Autodesk Inventor part; units mm, degrees
ref_plane "Work Plane1" through (29, 0, 0) normal (0, -1, 0) x (1, 0, 0)
ref_plane "YZ Plane" through (0, 0, 0) normal (1, 0, 0) x (0, 1, 0)
ref_plane "XZ Plane" through (0, 0, 0) normal (0, 1, 0) x (-1, 0, 0)
sketch "Sketch1" plane through (0, 0, 0) normal (0, 0, 1) x (1, 0, 0)
  line L0 (-0.5, 0) -> (6, 0)
  line L1 (6, 0) -> (6, 1)
  line L2 (6, 1) -> (1, 1)
  line L3 (1, 1) -> (0.7545, 1)
  line L4 (0.7545, 1) -> (0, 1)
  line L5 (0, 1) -> (0, 1.9)
  line L6 (0, 1.9) -> (-2, 1.9)
  line L7 (-2, 1.9) -> (-2, 0.866)
  line L8 (-2, 0.866) -> (-1, 0.866)
  line L9 (-1, 0.866) -> (-0.5, 0)
  line L10 (-3.6, 0) -> (7.6, 0)
  line L11 (0, -0.38) -> (0, 2.28)
  line L12 (1, 1) -> (0, 1) construction
  dimension "d1" = 5
  dimension "d2" = 0.2455
  dimension "d3" = 2
  dimension "d4" = 1
  dimension "d5" = 60
  dimension "d6" = 2
  dimension "d7" = 2
  dimension "d8" = 1.7321
  dimension "d9" = 3.8
  dimension "d26" = 6
revolve "Body" add sketch "Sketch1" angle 360 about axis through (-0.5, 0, 0) along (1, 0, 0)
sketch "Sketch2" plane through (-2, 0, 0) normal (-1, 0, 0) x (0, 0, 1)
  circle A0 centre (0, 0) radius 0.866
  line L0 (0, -2.66) -> (0, 2.66)
  line L1 (-2.66, 0) -> (2.66, 0)
  line L2 (0.866, 0) -> (0.433, -0.75)
  line L3 (0.433, -0.75) -> (-0.433, -0.75)
  line L4 (-0.433, -0.75) -> (-0.866, 0)
  line L5 (-0.866, 0) -> (-0.433, 0.75)
  line L6 (-0.433, 0.75) -> (0.433, 0.75)
  line L7 (0.433, 0.75) -> (0.866, 0)
  point P0 (0, 0)
extrude "Slot" add sketch "Sketch2" against normal up to next contours L7 A0 | A0 L2 | L6 L0 A0 | A0 L0 L3 | L0 L6 A0 | A0 L3 L0 | L4 A0 | A0 L5
fillet "Fillet1" radius 0.2 1 edges at (-2, -1.9, 0)
thread "Thread"
chamfer "Chamfer1" distance 0.2454 distance2 0.2454 1 edges at (6, -1, 0) measured on face at (6, -0.4588, -0.3309)
ref_plane "Work Plane1" through (29, 0, 0) normal (0, -1, 0) x (1, 0, 0)
fillet "Fillet2" radius 0.1 1 edges at (0, -1, 0)
equation "\"d1\" = GEL"
equation "\"d3\" = KOH"
equation "\"d4\" = INTI"
equation "\"d6\" = GD"
equation "\"d7\" = BDM"
equation "\"d8\" = 1.1547 * SW"
equation "\"d9\" = KOD"
equation "\"d26\" = NLG"
equation "\"d30\" = R"
equation "\"d17\" = RR"
equation "\"d13\" = GEL"
equation "\"d15\" = -0.5 * SPD + 0.5 * GD"
equation "\"d16\" = GUL"
equation "\"GD\" = 2"
equation "\"NLG\" = 6"
equation "\"GEL\" = 5"
equation "\"KOD\" = 3.8"
equation "\"KOH\" = 2"
equation "\"INTI\" = 1"
equation "\"GAL\" = 0.61345 * PTC"
equation "\"GUL\" = 0.61345 * PTC"
equation "\"BDM\" = NND"
equation "\"SW\" = 1.5"
equation "\"RR\" = 0.2"
equation "\"SPD\" = NND - 1.2269 * PTC"
equation "\"R\" = 0.1"
equation "\"TOA\" = 30deg"
equation "\"GD1\" = THREADDIA - 1.2269 * PTC"
equation "\"THREADDIA\" = 2"
equation "\"FAWI\" = 45deg"
equation "\"PTC\" = 0.4"
equation "\"NND\" = 2"
equation "\"E0\" = 1.155 * SW"
properties part number "ISO 4762 - M2 x 6" material "Stainless Steel, 440C"
Could you check a few things on this model? Use its own coordinates, in mm. A direction names the side the tool comes from. Give positions to 0.01 mm unless a question says otherwise; leave off trailing zeros. Order: outer loops, then holes, each group sorted by start corner. A loop starts at its lowest first (then second) coordinate and runs counter-clockwise, first axis right, second up. Notation, with made-up numbers: (0, 31) -> (24, 31) arc R22 ccw to (24, 51) -> close; hole circle Ø3 at (31.25, -9). An arc over 180 degrees is marked (long way). Return JSON: item names as keys, results as strings.
1. For pin 1 Ø2 at (x, z) = (-0.5, -1.5) entering from +Y; pin 2 Ø1 at (x, z) = (4.5, -0.5) entering from -Y; pin 3 Ø1.5 at (x, z) = (1.5, 1.5) entering from -Y, each with a flat end and sliding along its axis, tell me the tip position at first contact or that it passes through.
Answer list:
{"pin 1": "stops at y = 1.83", "pin 2": "stops at y = -1", "pin 3": "stops at y = -0.66"}
2. Thinking about a two-plate mould opening in Z: for faces 1 (the flat face through (-1.5, -0.75, 0)), 2 (the flat face through (-2, 1, 0)), 3 (the cylindrical face through (-0.91, -1.9, -0.08)), which applies, pulls with the +Z half, pulls with the -Z half, needs draft (parallel to the pull), parting line crosses it, or undercut?
Answer list:
{"face 1": "undercut", "face 2": "needs draft", "face 3": "parting line crosses it"}
3. Imagine slicing it at A-A on x = 3. List the corners of the cut face in (y, z) for me, then the cut area to 3 significant figures.
Answer list:
{"outline": "circle Ø2 at (0, 0)", "area": "3.14 mm2"}
4. I need wall thicknesses on line 1 (X direction, y = 0, z = -1.7); line 2 (Y direction, x = 5.5, z = -0.5); line 3 (Z direction, x = -1, y = -0.3). Which ranges of each line are inside material? Lowest first, please. Write a range as from..to.
Answer list:
{"line 1": "x = -2..0", "line 2": "y = -0.87..0.87", "line 3": "z = -1.88..-0.69, 0.69..1.88"}
5. On a 3-axis mill with a long thin cutter (end or side, diameter ignored), from which of +Z, -Z, +X, -X, +Y, -Y can I reach the whole of each face in a straight line? I mean faces 4 (the flat face through (0, 1, -1)), 5 (the flat face through (-1.5, 0.75, 0)), 6 (the flat face through (6, 0, 0)). Say none if no direction works.
Answer list:
{"face 4": "+X", "face 5": "-X", "face 6": "+Z, -Z, +X, +Y, -Y"}
